```python
from build123d import *

# Parameters (mm, degrees)
SKIZZE1_W                       = 70
SKIZZE1_H                       = 140
AUFSATZ_LINEAR_AUSTRAGEN1_DEPTH = 2
SKIZZE2_W                       = 25
SKIZZE2_H                       = 15
AUFSATZ_LINEAR_AUSTRAGEN2_DEPTH = 13
SCHNITT_LINEAR_AUSTRAGEN1_DEPTH = 146.086181285


with BuildPart() as part:
    # Skizze1 → Aufsatz-Linear austragen1 (new body)
    with BuildSketch(Plane(origin=(0, 0, 0), x_dir=(1, 0, 0), z_dir=(0, 1, 0))):
        Rectangle(SKIZZE1_W, SKIZZE1_H)
    extrude(amount=AUFSATZ_LINEAR_AUSTRAGEN1_DEPTH)

    # Skizze2 → Aufsatz-Linear austragen2 (add)
    with BuildSketch(Plane(origin=(0, 2, 0), x_dir=(1, 0, 0), z_dir=(0, 1, 0))):
        with Locations((-22.5, 62.5)):
            Rectangle(SKIZZE2_W, SKIZZE2_H)
        with Locations((-22.5, -62.5)):
            Rectangle(SKIZZE2_W, SKIZZE2_H)
    extrude(amount=AUFSATZ_LINEAR_AUSTRAGEN2_DEPTH)

    # Skizze3 → Schnitt-Linear austragen1 (cut, through all)
    with BuildSketch(Plane.XY.offset(70)):
        Polygon((-35, 15), (-35, 9.198729811), (-31.650635095, 15), align=None)
        Polygon((-14.330127019, 15), (-20.392304845, 4.5), (-16.062177826, 2), (-10, 12.5), (-10, 15), align=None)
    extrude(amount=-SCHNITT_LINEAR_AUSTRAGEN1_DEPTH, mode=Mode.SUBTRACT)


solid = part.part
```
Build history of the part. All positions in model axes, mm. A direction names the side the tool comes from. Give positions to 0.01 mm unless a question says otherwise; leave off trailing zeros. Loops run counter-clockwise (first coordinate to the right, second up) from the corner with the lowest first, then second, coordinate; pieces in that order, holes last.
1) 3-axis set-ups, long thin cutter, end or side, ignore diameter. For faces 1 (the face through (-12, 5, -55)), 2 (the face through (-35, 1, 1)), 3 (the face through (-17.32, 9.82, -62.4)), 4 (the face through (-10, 7, 63)): which of +Z, -Z, +X, -X, +Y, -Y reach the whole face in a straight line?
Values follow:
face 1: +X, -X, +Y
face 2: +Z, -Z, -X, +Y, -Y
face 3: +Z, -Z
face 4: +Z, -Z, +X, +Y
2) Drop a flat-ended pin along its axis: P1, Ø3, axis at y = 6, z = 61.5, coming from the +X side. Give the stop position or say it passes through.
Values follow:
P1: stops at x = -10
3) Band-saw the part on B-B on y = 7.25. List the corners of the cut face in (x, z), then the cut area to 3 significant figures.
Values follow:
outline: (-35, -70) - (-18.8, -70) - (-18.8, -55) - (-35, -55) - close; (-35, 55) - (-18.8, 55) - (-18.8, 70) - (-35, 70) - close; (-13.03, -70) - (-10, -70) - (-10, -55) - (-13.03, -55) - close; (-13.03, 55) - (-10, 55) - (-10, 70) - (-13.03, 70) - close
area: 577 mm2
4) Band-saw the part on D-D on x = -12. List the corners of the cut face in (y, z), then the cut area to 3 significant figures.
Values follow:
outline: (0, -70) - (9.04, -70) - (9.04, -55) - (2, -55) - (2, 55) - (9.04, 55) - (9.04, 70) - (0, 70) - close
area: 491 mm2
5) Band-saw the part on C-C on z = 53. List the corners of the cut face in (x, y).
Values follow:
outline: (-35, 0) - (35, 0) - (35, 2) - (-35, 2) - close
6) Probe line 1 along Z through (x, y) = (-22, 5.75); line 2 along Y through (x, z) = (31, 18); line 3 along X through (y, z) = (4.75, 57). List the from-to ranges inside material, lowest first.
Values follow:
line 1: z = -70 to -55, 55 to 70
line 2: y = 0 to 2
line 3: x = -35 to -20.25, -14.47 to -10
7) Band-saw the part on A-A on x = -29. List the corners of the cut face in (y, z), then the cut area to 3 significant figures.
Values follow:
outline: (0, -70) - (15, -70) - (15, -55) - (2, -55) - (2, 55) - (15, 55) - (15, 70) - (0, 70) - close
area: 670 mm2
8) Two-plate mould, pull along X, no slides. Class faces 5 (the face through (-17.32, 9.82, 62.6)), 6 (the face through (0, 0, -1)), 7 (the face through (-18.26, 3.27, -62.4)), 8 (the face through (-33.35, 12.06, 62.6)): released by +X, released by -X, zero draft, split by the parting line, or undercut.
Values follow:
face 5: undercut
face 6: zero draft
face 7: undercut
face 8: released by -X
